Study the drawing (mm; zero at the part's minimum x, y, z) and answer. Round coordinates to 2 decimals unless told otherwise and drop trailing zeros. Loops run counter-clockwise (first coordinate to the right, second up) from the corner with the lowest first, then second, coordinate; pieces in that order, holes last. Notation, with made-up numbers: M 84,12.5 L 102,12.5 A14 cw 102,31.5 Z; hole C 6.25,50.25 d3. An arc over 180 degrees is marked long. Put each result on its own line as item: value. Start each with the question number.
(1) A flat-ended cylindrical pin translates along its axis: P1, Ø3, axis at x = 53.08, z = 55.9, coming from the -Y side. Find the tip coordinate at first contact, or state that the pin passes through.
(2) Straight lines are drawn through the part: line 1 (X direction, y = 2.75, z = 5.1); line 2 (Z direction, x = 53.08, y = 3); line 3 (Z direction, x = 4, y = 8). For each, find the intervals that lie inside material, in ascending order.
(3) Section A-A, the plane z = 55.9 is taken. Determine the outline of the cut face in (x, y), then the cut area to 3 significant figures.
(4) Determine the mould class of the marked faces 1, 2 and 3 for opening direction Z: released by +Z, released by -Z, zero draft, split by the parting line, or undercut.
(5) Section B-B, the plane x = 4.82 is taken. Determine the outline of the cut face in (y, z), then the cut area to 3 significant figures.
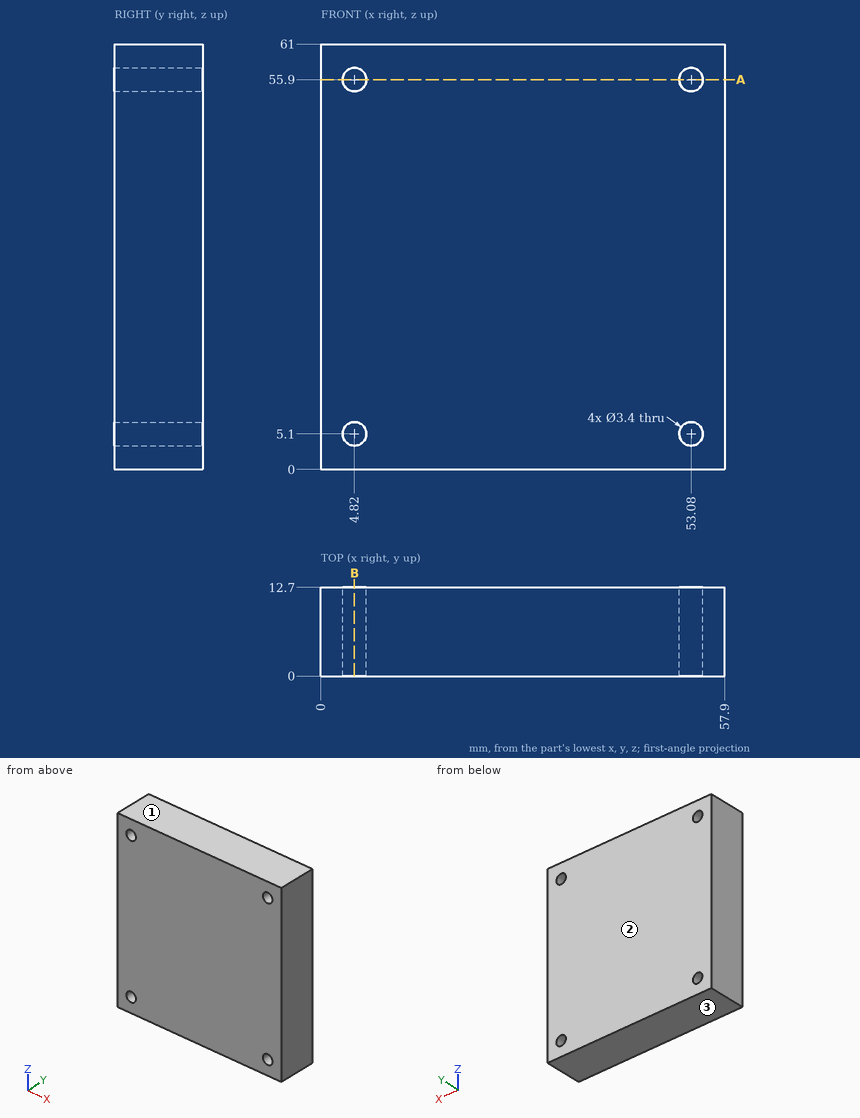
Recorded:
1. P1: passes through
2. line 1: x = 0 to 3.12, 6.52 to 51.38, 54.78 to 57.9
2. line 2: z = 0 to 3.4, 6.8 to 54.2, 57.6 to 61
2. line 3: z = 0 to 3.61, 6.59 to 54.41, 57.39 to 61
3. outline: M 0,0 L 3.12,0 L 3.12,12.7 L 0,12.7 Z; M 6.52,0 L 51.38,0 L 51.38,12.7 L 6.52,12.7 Z; M 54.78,0 L 57.9,0 L 57.9,12.7 L 54.78,12.7 Z
3. area: 649 mm²
4. face 1: released by +Z
4. face 2: zero draft
4. face 3: released by -Z
5. outline: M 0,0 L 12.7,0 L 12.7,3.4 L 0,3.4 Z; M 0,6.8 L 12.7,6.8 L 12.7,54.2 L 0,54.2 Z; M 0,57.6 L 12.7,57.6 L 12.7,61 L 0,61 Z
5. area: 688 mm²
